```python
from build123d import *

# Parameters (mm, degrees)
F0_W            = 203.2
F0_H            = 203.2
F1_DEPTH        = 12.7
F2_W            = 12.7
F2_H            = 101.6
F3_DEPTH        = 101.6
F4_R            = 50.79999
F5_R            = 8.73125
F6_DEPTH        = 25.4
F7_R            = 8.73125
F8_DEPTH        = 25.4
F8_COPIES_COUNT = 4


# Not quite as in the source:
# - a fillet or chamfer is up to 0.001 mm smaller than in the source, because OpenCascade refuses the exact size
# - a pattern or mirror of a feature is missing from the dataset's text; its kind, count and spacing are read off the source's solid


with BuildPart() as f1:
    # F0 (on Front) → F1 (new body)
    with BuildSketch(Plane.XZ):
        Rectangle(F0_W, F0_H)
    extrude(amount=F1_DEPTH)

    # F2 (on face) → F3 (join)
    with BuildSketch(Plane.XZ.offset(12.7)):
        Rectangle(F2_W, F2_H)
    extrude(amount=F3_DEPTH)

    # F4 (radius 50.8 in the source; OpenCascade refuses exactly that, so slightly less here)
    f4_edges = [f1.edges().sort_by_distance(p)[0] for p in [
        (0, -114.3, 50.8),
        (0, -114.3, -50.8),
    ]]
    fillet(f4_edges, radius=F4_R)

    # F5 (on face) → F6 (cut)
    with BuildSketch(Plane.YZ.offset(6.35)):
        with Locations((-63.5, 0)):
            Circle(F5_R)
    extrude(amount=-F6_DEPTH, mode=Mode.SUBTRACT)

    # F7 (on face) → F8 (cut)
    with BuildSketch(Plane.XZ.offset(12.7)):
        with Locations((-63.5, 63.5)):
            Circle(F7_R)
    f8 = extrude(amount=-F8_DEPTH, mode=Mode.SUBTRACT)

    # F8_copies: F8 ×4 about axis
    f8_copies_axis = Axis((0, 0, 0), (0, 1, 0))
    for i in range(1, F8_COPIES_COUNT):
        add(f8.rotate(f8_copies_axis, i * 360 / F8_COPIES_COUNT), mode=Mode.SUBTRACT)


solid = f1.part
```
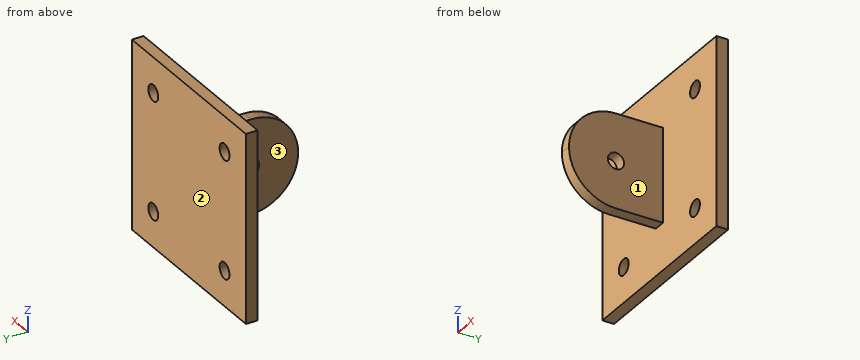
The model under review builds one solid part; all positions refer to its coordinate system, in mm. Face numbers are marked on the shaded views. A direction names the side the tool comes from. Round coordinates to 2 decimals unless told otherwise and drop trailing zeros. Write each loop counter-clockwise with the first axis right and the second up, starting at its lowest first coordinate (ties: lowest second). Pieces come first, ordered by that corner, then holes. Notation, with made-up numbers: (27, 81) -> (58, 81) arc R8 ccw to (58, 86) -> close; hole circle Ø4 at (14, -26.5). An arc over 180 degrees is marked (long way). Use CSV: the item, a comma, the result in double quotes.
Q1. Consider section B-B (z = -63.5). Give the boundary of the cut face in (x, y).
Checks:
outline,"(-101.6, -12.7) -> (-72.23, -12.7) -> (-72.23, 0) -> (-101.6, 0) -> close; (-54.77, -12.7) -> (54.77, -12.7) -> (54.77, 0) -> (-54.77, 0) -> close; (72.23, -12.7) -> (101.6, -12.7) -> (101.6, 0) -> (72.23, 0) -> close"
Q2. Consider section A-A (x = -63.5). Give the boundary of the cut face in (y, z).
Checks:
outline,"(-12.7, -101.6) -> (0, -101.6) -> (0, -72.23) -> (-12.7, -72.23) -> close; (-12.7, -54.77) -> (0, -54.77) -> (0, 54.77) -> (-12.7, 54.77) -> close; (-12.7, 72.23) -> (0, 72.23) -> (0, 101.6) -> (-12.7, 101.6) -> close"
Q3. Consider section D-D (z = 30). Give the boundary of the cut face in (x, y).
Checks:
outline,"(-101.6, -12.7) -> (-6.35, -12.7) -> (-6.35, -104.5) -> (6.35, -104.5) -> (6.35, -12.7) -> (101.6, -12.7) -> (101.6, 0) -> (-101.6, 0) -> close"
Q4. Consider section C-C (y = -7.5). Give the boundary of the cut face in (x, z).
Checks:
outline,"(-101.6, -101.6) -> (101.6, -101.6) -> (101.6, 101.6) -> (-101.6, 101.6) -> close; hole circle Ø17.46 at (-63.5, -63.5); hole circle Ø17.46 at (-63.5, 63.5); hole circle Ø17.46 at (63.5, -63.5); hole circle Ø17.46 at (63.5, 63.5)"
Q5. For pin 1 Ø1 at (x, z) = (34, 9.5) entering from -Y; pin 2 Ø1 at (y, z) = (-21, 50.5) entering from -X; pin 3 Ø14 at (x, y) = (3, -30.5) entering from -Z, all flat-tipped, find the tip position at first contact; note any pin that passes through.
Checks:
pin 1,"y = -12.7"
pin 2,"x = -6.35"
pin 3,"z = -50.8"
Q6. To check wall thickness, follow probe 1 along Z at (x, y) = (-63, -5); probe 2 along Z at (x, y) = (-3.75, -63.5). State the ranges of each line that lie inside material, in increasing order. Write a range as [from, to].
Checks:
probe 1,"[-101.6, -72.22], [-54.78, 54.78], [72.22, 101.6]"
probe 2,"[-50.8, -8.73], [8.73, 50.8]"
Q7. For the marked faces 1, 2 and 3, list the 3-axis set-ups (+Z, -Z, +X, -X, +Y, -Y) from which the entire face can be reached by the end or side of a thin tool; tool diameter is ignored.
Checks:
face 1,"+Z, -Z, +X, -Y"
face 2,"+Z, -Z, +X, -X, +Y"
face 3,"+Z, -Z, -X, -Y"
